Part model, mm, in its own coordinate system. Face numbers are marked on the shaded views. A direction names the side the tool comes from. Coordinates: 2 decimals unless noted, no trailing zeros. Loops run counter-clockwise (first coordinate to the right, second up) from the corner with the lowest first, then second, coordinate; pieces in that order, holes last. Notation, with made-up numbers: (37, 64) -> (42, 64) arc R19 ccw to (42, 78) -> close; hole circle Ø7 at (85.25, 46). An arc over 180 degrees is marked (long way). One line per question, with ' | ' between items. Start each with the question number.
1) Probe L1, parallel to Y at x = -221, z = 397; L2, parallel to X at y = 338.5, z = 77; L3, parallel to Z at x = -205.5, y = 760. List the from-to ranges inside material, lowest first. Write a range as from..to.
2) Two-plate mould, pull along Y, no slides. Class the marked faces 3, 4, 5 and 6: released by +Y, released by -Y, zero draft, split by the parting line, or undercut.
3) 3-axis set-ups, long thin cutter, end or side, ignore diameter. For the marked faces 1 and 2: which of +Z, -Z, +X, -X, +Y, -Y reach the whole face in a straight line?
4) Drop flat-ended pins along their axis: pin 1 (2 mm diameter, centred on x = 30.5, y = 712, fed in from -Z); pin 2 (8 mm diameter, centred on x = -201.5, y = -614, fed in from -Z). Give the stop position or say it passes through.
5) Cut at B-B (z = 59.5). Count the separate pieces of the cut face and the enclosed holes in it, plus the area to 3 significant figures.
6) Cut at A-A (x = 167). List the corners of the cut face in (y, z).
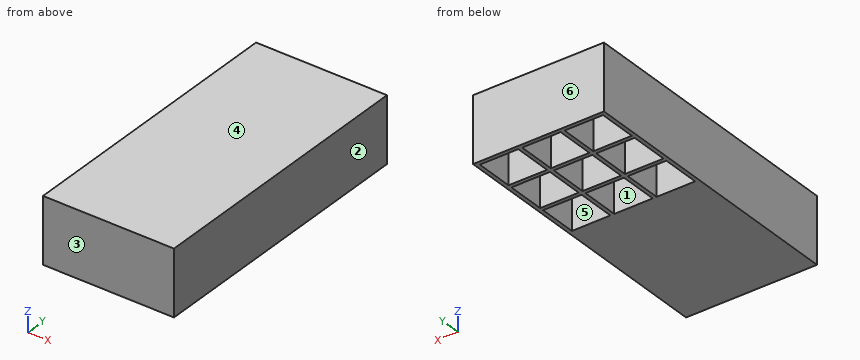
from build123d import *

# Parameters (mm, degrees)
SKETCH1_W           = 850
SKETCH1_H           = 1850
SKETCH1_W_2         = 250
SKETCH1_H_2         = 250
BOSS_EXTRUDE1_DEPTH = 400
SKETCH2_W           = 850
SKETCH2_H           = 1850
BOSS_EXTRUDE2_DEPTH = 25


with BuildPart() as part:
    # Sketch1 → Boss-Extrude1 (new body)
    with BuildSketch(Plane.XY):
        Rectangle(SKETCH1_W, SKETCH1_H)
        with Locations((275, 500)):
            Rectangle(SKETCH1_W_2, SKETCH1_H_2, mode=Mode.SUBTRACT)
        with Locations((275, 775)):
            Rectangle(SKETCH1_W_2, SKETCH1_H_2, mode=Mode.SUBTRACT)
        with Locations((0, 775)):
            Rectangle(SKETCH1_W_2, SKETCH1_H_2, mode=Mode.SUBTRACT)
        with Locations((-275, 775)):
            Rectangle(SKETCH1_W_2, SKETCH1_H_2, mode=Mode.SUBTRACT)
        with Locations((0, 500)):
            Rectangle(SKETCH1_W_2, SKETCH1_H_2, mode=Mode.SUBTRACT)
        with Locations((-275, 500)):
            Rectangle(SKETCH1_W_2, SKETCH1_H_2, mode=Mode.SUBTRACT)
        with Locations((275, 225)):
            Rectangle(SKETCH1_W_2, SKETCH1_H_2, mode=Mode.SUBTRACT)
        with Locations((0, 225)):
            Rectangle(SKETCH1_W_2, SKETCH1_H_2, mode=Mode.SUBTRACT)
        with Locations((-275, 225)):
            Rectangle(SKETCH1_W_2, SKETCH1_H_2, mode=Mode.SUBTRACT)
    extrude(amount=BOSS_EXTRUDE1_DEPTH)

    # Sketch2 → Boss-Extrude2 (add)
    with BuildSketch(Plane.XY.offset(400)):
        Rectangle(SKETCH2_W, SKETCH2_H)
    extrude(amount=BOSS_EXTRUDE2_DEPTH)


solid = part.part
Reported:
1) L1: y = -925..100, 350..375, 625..650, 900..925 | L2: x = -425..-400, -150..-125, 125..150, 400..425 | L3: z = 400..425
2) face 3: released by -Y | face 4: zero draft | face 5: undercut | face 6: released by +Y
3) face 1: -Z | face 2: +Z, -Z, +X, +Y, -Y
4) pin 1: stops at z = 400 | pin 2: stops at z = 0
5) separate pieces: 1 | enclosed holes: 9 | area: 1,010,000 mm²
6) outline: (-925, 0) -> (100, 0) -> (100, 400) -> (350, 400) -> (350, 0) -> (375, 0) -> (375, 400) -> (625, 400) -> (625, 0) -> (650, 0) -> (650, 400) -> (900, 400) -> (900, 0) -> (925, 0) -> (925, 425) -> (-925, 425) -> close
